```python
from build123d import *

# Parameters (mm, degrees)
BOSS_EXTRUDE1_DEPTH = 42
SKETCH2_W           = 20
SKETCH2_H           = 20
CUT_EXTRUDE1_DEPTH  = 112.610931364
CUT_EXTRUDE2_DEPTH  = 37
SKETCH6_R           = 2.6
CUT_EXTRUDE4_DEPTH  = 106.721331812
SKETCH5_R           = 2.6
CUT_EXTRUDE3_DEPTH  = 6
BOSS_EXTRUDE2_DEPTH = 17
SKETCH7_R           = 12.5
CUT_EXTRUDE5_DEPTH  = 110.827136902
BOSS_EXTRUDE4_DEPTH = 17
SKETCH12_R          = 1.6
CUT_EXTRUDE6_DEPTH  = 112.610931364


with BuildPart() as part:
    # Sketch1 → Boss-Extrude1 (new body)
    with BuildSketch(Plane(origin=(0, 0, 0), x_dir=(1, 0, 0), z_dir=(0, 1, 0))):
        Polygon((0, 0), (0, 82), (26, 82), (63, 67), (63, 15), (26, 0), align=None)
    extrude(amount=BOSS_EXTRUDE1_DEPTH)

    # Sketch2 → Cut-Extrude1 (cut, through all)
    with BuildSketch(Plane.XY):
        with Locations((10, 32)):
            Rectangle(SKETCH2_W, SKETCH2_H)
    extrude(amount=-CUT_EXTRUDE1_DEPTH, mode=Mode.SUBTRACT)

    # Sketch3 → Cut-Extrude2 (cut)
    with BuildSketch(Plane(origin=(0, 42, 0), x_dir=(1, 0, 0), z_dir=(0, 1, 0))):
        Polygon((26, 82), (26, 62), (20, 62), (20, 20), (26, 20), (26, 0), (63, 15), (63, 67), align=None)
    extrude(amount=-CUT_EXTRUDE2_DEPTH, mode=Mode.SUBTRACT)

    # Sketch6 → Cut-Extrude4 (cut, through all)
    with BuildSketch(Plane(origin=(0, 22, 0), x_dir=(1, 0, 0), z_dir=(0, 1, 0))):
        with Locations(Location((10, 72, 0), (0, 0, 270))):
            Circle(SKETCH6_R)
        with Locations(Location((10, 41, 0), (0, 0, 270))):
            Circle(SKETCH6_R)
        with Locations(Location((10, 10, 0), (0, 0, 270))):
            Circle(SKETCH6_R)
    extrude(amount=-CUT_EXTRUDE4_DEPTH, mode=Mode.SUBTRACT)

    # Sketch5 → Cut-Extrude3 (cut)
    with BuildSketch(Plane.ZY.offset(-20)):
        with Locations(Location((-72, 32, 0), (0, 0, 270))):
            Circle(SKETCH5_R)
        with Locations(Location((-10, 32, 0), (0, 0, 270))):
            Circle(SKETCH5_R)
    extrude(amount=-CUT_EXTRUDE3_DEPTH, mode=Mode.SUBTRACT)

    # Sketch4 → Boss-Extrude2 (add)
    with BuildSketch(Plane(origin=(0, 5, 0), x_dir=(1, 0, 0), z_dir=(0, 1, 0))):
        Polygon((26, 20), (63, 20), (63, 15), (26, 0), align=None)
    extrude(amount=BOSS_EXTRUDE2_DEPTH)

    # Sketch7 → Cut-Extrude5 (cut, through all)
    with BuildSketch(Plane(origin=(0, 5, 0), x_dir=(1, 0, 0), z_dir=(0, 1, 0))):
        with Locations(Location((39, 41, 0), (0, 0, 270))):
            Circle(SKETCH7_R)
    extrude(amount=-CUT_EXTRUDE5_DEPTH, mode=Mode.SUBTRACT)

    # Sketch10 → Boss-Extrude4 (add)
    with BuildSketch(Plane(origin=(0, 5, 0), x_dir=(1, 0, 0), z_dir=(0, 1, 0))):
        with BuildLine():
            Line((26, 62), (26, 41))
            ThreePointArc((26, 41), (39, 28), (52, 41))
            Line((52, 41), (52, 71.459459459))
            Line((52, 71.459459459), (63, 67))
            Line((63, 67), (63, 20))
            Line((63, 20), (20, 20))
            Line((20, 20), (20, 62))
            Line((20, 62), (26, 62))
        make_face()
    extrude(amount=BOSS_EXTRUDE4_DEPTH)

    # Sketch12 → Cut-Extrude6 (cut, through all)
    with BuildSketch(Plane.XZ):
        with Locations(Location((23.5, -25.5, 0), (0, 0, 270))):
            Circle(SKETCH12_R)
        with Locations(Location((54.5, -25.5, 0), (0, 0, 270))):
            Circle(SKETCH12_R)
        with Locations(Location((54.5, -56.5, 0), (0, 0, 270))):
            Circle(SKETCH12_R)
        with Locations(Location((23.5, -56.5, 0), (0, 0, 270))):
            Circle(SKETCH12_R)
    extrude(amount=-CUT_EXTRUDE6_DEPTH, mode=Mode.SUBTRACT)


solid = part.part
```
Input: part model. Units: mm. Frame: model coordinates. A direction names the side the tool comes from. Give positions to 0.01 mm unless a question says otherwise; leave off trailing zeros. Order: outer loops, then holes, each group sorted by start corner. A loop starts at its lowest first (then second) coordinate and runs counter-clockwise, first axis right, second up. Notation, with made-up numbers: (20, 66.5) -> (30, 66.5) arc R13 cw to (30, 87.5) -> close; hole circle Ø4 at (42, 28.5). An arc over 180 degrees is marked (long way). Write each question's results on one line, items separated by ' | '. Start each with the question number.
Item 1: Mould query, pull axis Z, two halves, no side actions, for faces 1 (the flat face through (16, 16, 0)), 2 (the cylindrical face through (7.693, 11.154, -8.8)), 3 (the flat face through (63, 11, -41)). Classes: pulls with the +Z half, pulls with the -Z half, needs draft (parallel to the pull), parting line crosses it, or undercut.
Item 2: Cut plane B-B on y = 32. Return the cut outline in (x, z), then the cut area to 3 significant figures.
Item 3: Set-up query: faces 4 (the flat face through (26, 19, -66)), 5 (the flat face through (20, 30, -8)), 6 (the flat face through (23, 32, -20)). Return all of +Z, -Z, +X, -X, +Y, -Y with unobstructed straight access to the full face (end or side cutting, diameter ignored); none if empty.
Item 4: Cut plane C-C on x = 10. Return the cut outline in (y, z).
Item 5: Contact query for flat-ended pins moving along their axis: P1, Ø3, axis at x = 34.5, y = 18, coming from the +Z side; P2, Ø1.5, axis at x = 28, y = 13, coming from the -Z side; P3, Ø1, axis at x = 52, y = 17, coming from the -Z side; P4, Ø1.8, axis at x = 23, y = 27, coming from the +Z side. Output: stop coordinate, or through.
Item 6: Line query: line 1 (Z direction, x = 22, y = 32); line 2 (X direction, y = 15, z = -25.5); line 3 (X direction, y = 10, z = -41). Output: solid intervals per line, ascending.
Item 7: Cut plane A-A on z = -56.5. Return the cut outline in (x, y), then the cut area to 3 significant figures.
Item 8: Cut plane D-D on z = -76. Return the cut outline in (x, y), then the cut area to 3 significant figures.
Established:
1) face 1: pulls with the +Z half | face 2: undercut | face 3: needs draft
2) outline: (20, -82) -> (26, -82) -> (26, -74.6) -> (20, -74.6) -> close; (20, -69.4) -> (26, -69.4) -> (26, -62) -> (20, -62) -> close; (20, -20) -> (26, -20) -> (26, -12.6) -> (20, -12.6) -> close; (20, -7.4) -> (26, -7.4) -> (26, 0) -> (20, 0) -> close | area: 178 mm^2
3) face 4: -Z, +Y | face 5: +Z, -Z, -X, +Y | face 6: +X, -X, +Y
4) outline: (0, -82) -> (22, -82) -> (22, -74.6) -> (0, -74.6) -> close; (0, -69.4) -> (22, -69.4) -> (22, -43.6) -> (0, -43.6) -> close; (0, -38.4) -> (22, -38.4) -> (22, -12.6) -> (0, -12.6) -> close; (0, -7.4) -> (22, -7.4) -> (22, 0) -> (0, 0) -> close
5) P1: z = -2.84 | P2: z = -35.44 | P3: z = -71.46 | P4: z = 0
6) line 1: -82 to -74.6, -69.4 to -62, -20 to -12.6, -7.4 to 0 | line 2: 0 to 21.9, 25.1 to 52.9, 56.1 to 63 | line 3: 0 to 7.4, 12.6 to 26, 52 to 63
7) outline: (0, 0) -> (21.9, 0) -> (21.9, 22) -> (0, 22) -> close; (25.1, 0) -> (52.9, 0) -> (52.9, 22) -> (52, 22) -> (52, 5) -> (26, 5) -> (26, 22) -> (25.1, 22) -> close; (56.1, 0) -> (63, 0) -> (63, 22) -> (56.1, 22) -> close | area: 803 mm^2
8) outline: (0, 0) -> (40.8, 0) -> (40.8, 5) -> (26, 5) -> (26, 42) -> (20, 42) -> (20, 22) -> (0, 22) -> close | area: 766 mm^2
